CAD build for the part. Positions are in the model's coordinates, mm. A direction names the side the tool comes from. Coordinates: 2 decimals unless noted, no trailing zeros. Loops run counter-clockwise (first coordinate to the right, second up) from the corner with the lowest first, then second, coordinate; pieces in that order, holes last. Notation, with made-up numbers: (7.25, 67) -> (57.25, 67) arc R16 cw to (57.25, 97) -> close; hole circle Ø7 at (51.25, 52). An arc over 180 degrees is marked (long way). Write item = value, one per line. Start each with the question number.
(1) Pull direction Y, two halves, no side cores. Call faces 5 (the face through (-1.4, -26, 5)), 6 (the face through (1.78, -15.9, 4.93)), 7 (the face through (0.714, 17.185, 4.93)): +Y half, -Y half, draft (parallel to the pull), parting line (faces both ways), or undercut.
(2) Flat gauge pins, fed straight in: P1, Ø1.5, axis at x = 8, z = 6.5, coming from the -Y side; P2, Ø5, axis at y = -26, z = 4.5, coming from the +X side; P3, Ø2, axis at x = -13, z = 1.5, coming from the +Y side. Where does each tip first touch, or does it go through?
(3) Band-saw the part on B-B (z = 4). Write the cut outline in (x, y), and give its area (3 significant figures).
(4) Drill centre lines: line 1 (X direction, y = -18, z = 9); line 2 (X direction, y = 0, z = 7.5); line 3 (Y direction, x = 8.5, z = 5.25). Where is each one in solid material? Low to high. Write a range as from..to.
(5) Band-saw the part on D-D (x = -9). Write the cut outline in (y, z), and give its area (3 significant figures).
(6) Band-saw the part on A-A (y = -21). Write the cut outline in (x, z).
(7) Tool access for faces 1 (the face through (-1.764, -15.92, 4.93)), 2 (the face through (1.4, -26, 5)), 3 (the face through (3, -26, 5)), 4 (the face through (-3, -26, 5)): list every direction of +Z, -Z, +X, -X, +Y, -Y with a clear straight run to the whole face (end or side of a thin tool).
(8) Band-saw the part on C-C (y = -28.5). Write the cut outline in (x, z), and give its area (3 significant figures).
```python
from build123d import *

# Parameters (mm, degrees)
F1_DEPTH = 10
F2_R     = 2
F3_DEPTH = 30


with BuildPart() as f1:
    # F0 (on Top) → F1 (new body)
    with BuildSketch(Plane.XY):
        with BuildLine():
            ThreePointArc((-2.72093, -15.360877), (0, 15.6), (2.72093, -15.360877))
            ThreePointArc((2.72093, -15.360877), (1.773927, -15.908371), (1.4, -16.936351))
            Line((1.4, -16.936351), (1.4, -34.936351))
            Line((1.4, -34.936351), (3, -34.936351))
            Line((3, -34.936351), (3, -16.936351))
            ThreePointArc((3, -16.936351), (0, 17.2), (-3, -16.936351))
            Line((-3, -16.936351), (-3, -34.936351))
            Line((-3, -34.936351), (-1.4, -34.936351))
            Line((-1.4, -34.936351), (-1.4, -16.936351))
            ThreePointArc((-1.4, -16.936351), (-1.773927, -15.908371), (-2.72093, -15.360877))
        make_face()
    extrude(amount=F1_DEPTH)

    # F2 (on face) → F3 (cut)
    with BuildSketch(Plane.YZ.offset(3)):
        with Locations((-28.936351, 5)):
            Circle(F2_R)
    extrude(amount=-F3_DEPTH, mode=Mode.SUBTRACT)


solid = f1.part
```
Findings below:
q1.face_5 = draft
q1.face_6 = undercut
q1.face_7 = parting line
q2.P1 = -15.6
q2.P2 = 3
q2.P3 = 12.32
q3.outline = (-3, -34.94) -> (-1.4, -34.94) -> (-1.4, -30.67) -> (-3, -30.67) -> close; (-3, -27.2) -> (-1.4, -27.2) -> (-1.4, -16.94) arc R1.6 ccw to (-2.72, -15.36) arc R15.6 cw (long way) to (2.72, -15.36) arc R1.6 ccw to (1.4, -16.94) -> (1.4, -27.2) -> (3, -27.2) -> (3, -16.94) arc R17.2 ccw (long way) to (-3, -16.94) -> close; (1.4, -34.94) -> (3, -34.94) -> (3, -30.67) -> (1.4, -30.67) -> close
q3.area = 206 mm²
q4.line_1 = -3..-1.4, 1.4..3
q4.line_2 = -17.2..-15.6, 15.6..17.2
q4.line_3 = -14.95..-13.08, 13.08..14.95
q5.outline = (-14.66, 0) -> (-12.74, 0) -> (-12.74, 10) -> (-14.66, 10) -> close; (12.74, 0) -> (14.66, 0) -> (14.66, 10) -> (12.74, 10) -> close
q5.area = 38.3 mm²
q6.outline = (-3, 0) -> (-1.4, 0) -> (-1.4, 10) -> (-3, 10) -> close; (1.4, 0) -> (3, 0) -> (3, 10) -> (1.4, 10) -> close
q7.face_1 = +Z, -Z
q7.face_2 = +Z, -Z, -Y
q7.face_3 = +Z, -Z, +X, -Y
q7.face_4 = +Z, -Z, -X, -Y
q8.outline = (-3, 0) -> (-1.4, 0) -> (-1.4, 3.05) -> (-3, 3.05) -> close; (-3, 6.95) -> (-1.4, 6.95) -> (-1.4, 10) -> (-3, 10) -> close; (1.4, 0) -> (3, 0) -> (3, 3.05) -> (1.4, 3.05) -> close; (1.4, 6.95) -> (3, 6.95) -> (3, 10) -> (1.4, 10) -> close
q8.area = 19.5 mm²
